The listing builds one solid part. Answer for the finished solid, in the listing's coordinates (mm). A direction names the side the tool comes from. Coordinates: 2 decimals unless noted, no trailing zeros. Order: outer loops, then holes, each group sorted by start corner. A loop starts at its lowest first (then second) coordinate and runs counter-clockwise, first axis right, second up.
```python
from build123d import *

# Parameters (mm, degrees)
F1_DEPTH = 25
F2_R     = 2
F3_R     = 2
F4_R     = 1
F5_R     = 0.5


with BuildPart() as f1:
    # F0 (on Front) → F1 (new body)
    with BuildSketch(Plane.XZ):
        Polygon((-13.5, -15.483479), (-13.5, -6.983479), (7.5, -6.983479), (7.5, -15.483479), (6.3, -15.483479), (7.5, -17.083479), (10, -17.083479), (10, -4.083479), (3, -4.083479), (3, 5.916521), (0, 5.916521), (0, -4.083479), (-6, -4.083479), (-6, 5.916521), (-9, 5.916521), (-9, -4.083479), (-16, -4.083479), (-16, -17.083479), (-13.5, -17.083479), (-12.3, -15.483479), align=None)
    extrude(amount=F1_DEPTH)

    # F2
    f2_edges = [f1.edges().sort_by_distance(p)[0] for p in [
        (-13.5, -12.5, -6.983479),
        (7.5, -12.5, -6.983479),
    ]]
    fillet(f2_edges, radius=F2_R)

    # F3
    f3_edges = [f1.edges().sort_by_distance(p)[0] for p in [
        (10, -12.5, -4.083479),
        (-16, -12.5, -4.083479),
    ]]
    fillet(f3_edges, radius=F3_R)

    # F4
    f4_edges = [f1.edges().sort_by_distance(p)[0] for p in [
        (-6, -12.5, 5.916521),
        (0, -12.5, 5.916521),
    ]]
    fillet(f4_edges, radius=F4_R)

    # F5
    f5_edges = [f1.edges().sort_by_distance(p)[0] for p in [
        (10, -12.5, -17.083479),
        (-16, -12.5, -17.083479),
    ]]
    fillet(f5_edges, radius=F5_R)


solid = f1.part
```
1) A cutting plane is placed at A-A, the plane z = 2. Write down the section's boundary in (x, y), plus the area to 3 significant figures.
2) Straight lines are drawn through the part: probe 1 along X at (y, z) = (-6.25, -9.75); probe 2 along X at (y, z) = (-17.5, 2); probe 3 along Z at (x, y) = (5, -15). For each, find the intervals that lie inside material, in ascending order.
3) A cutting plane is placed at C-C, the plane x = 4.5. Write down the section's boundary in (y, z), plus the area to 3 significant figures.
4) Each of these flat-tipped pins is pushed along its axis until it touches: P1, Ø2.5, axis at x = -12.5, y = -16.5, coming from the +Z side; P2, Ø4.5, axis at y = -12.5, z = 1.5, coming from the +X side; P3, Ø5, axis at y = -17.5, z = 1, coming from the -X side. Where does it stop, or does it pass through?
5) A cutting plane is placed at D-D, the plane z = -14.5. Write down the section's boundary in (x, y).
6) For faces 1 (the flat face through (-12.908, -12.325, -16.295)), 2 (the flat face through (-9, -12, 1)), 3 (the flat face through (7.5, -12, -12)), 4 (the flat face through (-6, -12, 0)), 5 (the flat face through (6, -12, -4.083)), determine the directions among +Z, -Z, +X, -X, +Y, -Y from which every point of the face is accessible in a straight line to the end or side of a thin tool.
7) A cutting plane is placed at B-B, the plane y = -12.75. Write down the section's boundary in (x, z), plus the area to 3 significant figures.
8) The mould has two halves that part along Z. Classify faces 6 (the cylindrical face through (0.29, -12.68, 5.62)), 7 (the flat face through (10, -12, -11)), 8 (the cylindrical face through (6.899, -12.675, -7.554)): released by +Z, released by -Z, zero draft, split by the parting line, or undercut.
Working result:
1. outline: (-9, -25) - (-6, -25) - (-6, 0) - (-9, 0) - close; (0, -25) - (3, -25) - (3, 0) - (0, 0) - close
1. area: 150 mm2
2. probe 1: x = -16 to -13.5, 7.5 to 10
2. probe 2: x = -9 to -6, 0 to 3
2. probe 3: z = -6.98 to -4.08
3. outline: (-25, -6.98) - (0, -6.98) - (0, -4.08) - (-25, -4.08) - close
3. area: 72.5 mm2
4. P1: stops at z = -4.08
4. P2: stops at x = 3
4. P3: stops at x = -9
5. outline: (-16, -25) - (-13.5, -25) - (-13.5, 0) - (-16, 0) - close; (7.5, -25) - (10, -25) - (10, 0) - (7.5, 0) - close
6. face 1: -Z, +Y, -Y
6. face 2: +Z, -X, +Y, -Y
6. face 3: +Y, -Y
6. face 4: +Z, +Y, -Y
6. face 5: +Z, +X, +Y, -Y
7. outline: (-16, -16.58) arc R0.5 ccw to (-15.5, -17.08) - (-13.5, -17.08) - (-12.3, -15.48) - (-13.5, -15.48) - (-13.5, -8.98) arc R2 cw to (-11.5, -6.98) - (5.5, -6.98) arc R2 cw to (7.5, -8.98) - (7.5, -15.48) - (6.3, -15.48) - (7.5, -17.08) - (9.5, -17.08) arc R0.5 ccw to (10, -16.58) - (10, -6.08) arc R2 ccw to (8, -4.08) - (3, -4.08) - (3, 5.92) - (1, 5.92) arc R1 ccw to (0, 4.92) - (0, -4.08) - (-6, -4.08) - (-6, 4.92) arc R1 ccw to (-7, 5.92) - (-9, 5.92) - (-9, -4.08) - (-14, -4.08) arc R2 ccw to (-16, -6.08) - close
7. area: 187 mm2
8. face 6: released by +Z
8. face 7: zero draft
8. face 8: undercut
